```python
from build123d import *

# Parameters (mm, degrees)
SKETCH1_W           = 26.4
SKETCH1_H           = 32.8
BOSS_EXTRUDE1_DEPTH = 5
SKETCH2_W           = 26.4
SKETCH2_H           = 5
BOSS_EXTRUDE2_DEPTH = 30
SKETCH3_W           = 26.4
SKETCH3_H           = 5
BOSS_EXTRUDE3_DEPTH = 12.5
SKETCH4_W           = 26.4
SKETCH4_H           = 5
BOSS_EXTRUDE4_DEPTH = 60
SKETCH5_W           = 26.4
SKETCH5_H           = 5
BOSS_EXTRUDE5_DEPTH = 12.5
SKETCH6_W           = 26.4
SKETCH6_H           = 5
BOSS_EXTRUDE8_DEPTH = 5


with BuildPart() as part:
    # Sketch1 → Boss-Extrude1 (new body)
    with BuildSketch(Plane.XY):
        with Locations((-3.092887029, -2.09539749)):
            Rectangle(SKETCH1_W, SKETCH1_H)
    extrude(amount=BOSS_EXTRUDE1_DEPTH)

    # Sketch2 → Boss-Extrude2 (add)
    with BuildSketch(Plane.XY.offset(5)):
        with Locations((-3.092887029, 11.80460251)):
            Rectangle(SKETCH2_W, SKETCH2_H)
    extrude(amount=BOSS_EXTRUDE2_DEPTH)

    # Sketch3 → Boss-Extrude3 (add)
    with BuildSketch(Plane(origin=(0, 14.30460251, 0), x_dir=(1, 0, 0), z_dir=(0, 1, 0))):
        with Locations((-3.092887029, -32.5)):
            Rectangle(SKETCH3_W, SKETCH3_H)
    extrude(amount=BOSS_EXTRUDE3_DEPTH)

    # Sketch4 → Boss-Extrude4 (add)
    with BuildSketch(Plane(origin=(0, 0, 30), x_dir=(-1, 0, 0), z_dir=(0, 0, -1))):
        with Locations((3.092887029, 24.30460251)):
            Rectangle(SKETCH4_W, SKETCH4_H)
    extrude(amount=BOSS_EXTRUDE4_DEPTH)

    # Sketch5 → Boss-Extrude5 (add)
    with BuildSketch(Plane.XZ.offset(-21.80460251)):
        with Locations((-3.092887029, -27.5)):
            Rectangle(SKETCH5_W, SKETCH5_H)
    extrude(amount=BOSS_EXTRUDE5_DEPTH)

    # Sketch6 → Boss-Extrude8 (add)
    with BuildSketch(Plane.XY.offset(-25)):
        with Locations((-3.092887029, 11.80460251)):
            Rectangle(SKETCH6_W, SKETCH6_H)
    extrude(amount=BOSS_EXTRUDE8_DEPTH)


solid = part.part
```
Verification items for the finished model (mm, model axes). A direction names the side the tool comes from. Coordinates: 2 decimals unless noted, no trailing zeros. Loops run counter-clockwise (first coordinate to the right, second up) from the corner with the lowest first, then second, coordinate; pieces in that order, holes last. Notation, with made-up numbers: (83.25, -14) -> (105.25, -14) arc R14 ccw to (105.25, 10) -> close; hole circle Ø11 at (13.5, 21.25). An arc over 180 degrees is marked (long way). Answer in a Markdown table with one row per item.
1) Draft check along Z on faces 6 (the face through (-3, 21.805, 3)), 7 (the face through (-3, 18, -30)), 8 (the face through (-3, 18, 35)), 9 (the face through (-3, 18, -25)). Enter one of: released by +Z, released by -Z, zero draft, split by the parting line, or undercut.
The answers:
| item | result |
|---|---|
| face 6 | undercut |
| face 7 | released by -Z |
| face 8 | released by +Z |
| face 9 | undercut |
2) Scan lines: line 1 along Y through (x, z) = (-13, 1); line 2 along Z through (x, y) = (-6.25, -12); line 3 along Y through (x, z) = (-13.5, -2). Record each from-to range of solid material in increasing order. Write a range as from..to.
The answers:
| item | result |
|---|---|
| line 1 | y = -18.5..14.3, 21.8..26.8 |
| line 2 | z = 0..5 |
| line 3 | y = 21.8..26.8 |
3) Section check B-B (z = 22). Record the cut outline in (x, y).
The answers:
| item | result |
|---|---|
| outline | (-16.29, 9.3) -> (10.11, 9.3) -> (10.11, 14.3) -> (-16.29, 14.3) -> close; (-16.29, 21.8) -> (10.11, 21.8) -> (10.11, 26.8) -> (-16.29, 26.8) -> close |
4) Access from +Z, -Z, +X, -X, +Y, -Y to the whole of each face (thin tool, end or side, straight path). Record for faces 1 (the face through (-3, 14.305, -23)), 2 (the face through (-3, 26.805, 3)), 3 (the face through (-3, -4, 5)), 4 (the face through (-3, 12, -20)), 5 (the face through (-3, 9.305, -25)).
The answers:
| item | result |
|---|---|
| face 1 | +X, -X |
| face 2 | +Z, -Z, +X, -X, +Y |
| face 3 | +Z, +X, -X, -Y |
| face 4 | +X, -X, -Y |
| face 5 | -Z, +X, -X, -Y |
5) Section check D-D (z = -15). Record the cut outline in (x, y), and give its area (3 significant figures).
The answers:
| item | result |
|---|---|
| outline | (-16.29, 21.8) -> (10.11, 21.8) -> (10.11, 26.8) -> (-16.29, 26.8) -> close |
| area | 132 mm2 |
6) Section check A-A (y = 13). Record the cut outline in (x, z), and give its area (3 significant figures).
The answers:
| item | result |
|---|---|
| outline | (-16.29, -30) -> (10.11, -30) -> (10.11, -20) -> (-16.29, -20) -> close; (-16.29, 0) -> (10.11, 0) -> (10.11, 35) -> (-16.29, 35) -> close |
| area | 1,190 mm2 |
7) Depth check by flat-ended pin: P1, Ø1.5, axis at x = 6.5, z = -11.5, coming from the -Y side; P2, Ø3, axis at x = -9, y = 8.5, coming from the -Z side; P3, Ø12, axis at x = 4, y = -7.5, coming from the -Z side; P4, Ø8, axis at x = -1, z = 14.5, coming from the -Y side. Enter the tip coordinate at first touch or a pass-through.
The answers:
| item | result |
|---|---|
| P1 | stops at y = 21.8 |
| P2 | stops at z = -30 |
| P3 | stops at z = 0 |
| P4 | stops at y = 9.3 |
8) Section check C-C (x = 4.5). Record the cut outline in (y, z).
The answers:
| item | result |
|---|---|
| outline | (-18.5, 0) -> (14.3, 0) -> (14.3, 30) -> (21.8, 30) -> (21.8, -25) -> (14.3, -25) -> (14.3, -20) -> (9.3, -20) -> (9.3, -30) -> (26.8, -30) -> (26.8, 35) -> (9.3, 35) -> (9.3, 5) -> (-18.5, 5) -> close |
